from build123d import *

# Parameters (mm, degrees)
SKETCH1_W           = 19.05
SKETCH1_H           = 19.05
BOSS_EXTRUDE1_DEPTH = 19.05
SKETCH2_W           = 15.875
SKETCH2_H           = 15.875
BOSS_EXTRUDE2_DEPTH = 28.575
SKETCH3_W           = 15.875
SKETCH3_H           = 15.875
BOSS_EXTRUDE3_DEPTH = 28.575


with BuildPart() as part:
    # Sketch1 → Boss-Extrude1 (new body)
    with BuildSketch(Plane.XY):
        Rectangle(SKETCH1_W, SKETCH1_H)
    extrude(amount=BOSS_EXTRUDE1_DEPTH)

    # Sketch2 → Boss-Extrude2 (add)
    with BuildSketch(Plane(origin=(0, 9.525, 0), x_dir=(1, 0, 0), z_dir=(0, 1, 0))):
        with Locations((0, -9.525)):
            Rectangle(SKETCH2_W, SKETCH2_H)
    extrude(amount=BOSS_EXTRUDE2_DEPTH)

    # Sketch3 → Boss-Extrude3 (add)
    with BuildSketch(Plane(origin=(9.525, 0, 0), x_dir=(0, 0, -1), z_dir=(1, 0, 0))):
        with Locations((-9.525, 0)):
            Rectangle(SKETCH3_W, SKETCH3_H)
    extrude(amount=BOSS_EXTRUDE3_DEPTH)


solid = part.part
Geometry: final body of the model. Coordinates: model frame, mm. A direction names the side the tool comes from. Give positions to 0.01 mm unless a question says otherwise; leave off trailing zeros. Write each loop counter-clockwise with the first axis right and the second up, starting at its lowest first coordinate (ties: lowest second). Pieces come first, ordered by that corner, then holes.
(1) Access query for faces 1 (the flat face through (24, -7.938, 10)), 2 (the flat face through (24, 0, 17.462)), 3 (the flat face through (24, 7.938, 10)), 4 (the flat face through (0, 24, 17.462)). Directions: +Z, -Z, +X, -X, +Y, -Y. A direction counts if a zero-diameter tool reaches every point of the face in a straight line with its end or side. Return the directions, or none.
(2) Ray query, line 1 (X direction, y = 26.5, z = 12); line 2 (Z direction, x = -1.5, y = 29). Return the intervals inside material, ascending.
(3) Cut plane A-A, the plane z = 3. Return loops of the section in (x, y) (1 decimal).
(4) First-contact query: P1, Ø12.5, axis at x = -2.5, y = 17, coming from the -Z side; P2, Ø3, axis at y = 16.5, z = 3, coming from the -X side; P3, Ø4, axis at x = 29, y = -3.5, coming from the +Z side. Flat tips, straight axial feed; report the tip coordinate or a pass-through.
(5) Cut plane D-D, the plane x = 28. Return loops of the section in (y, z).
Values follow:
1. face 1: +Z, -Z, +X, -Y
1. face 2: +Z, +X, +Y, -Y
1. face 3: +Z, -Z, +X, +Y
1. face 4: +Z, +X, -X, +Y
2. line 1: x = -7.94 to 7.94
2. line 2: z = 1.59 to 17.46
3. outline: (-9.5, -9.5) - (9.5, -9.5) - (9.5, -7.9) - (38.1, -7.9) - (38.1, 7.9) - (9.5, 7.9) - (9.5, 9.5) - (7.9, 9.5) - (7.9, 38.1) - (-7.9, 38.1) - (-7.9, 9.5) - (-9.5, 9.5) - close
4. P1: stops at z = 1.59
4. P2: stops at x = -7.94
4. P3: stops at z = 17.46
5. outline: (-7.94, 1.59) - (7.94, 1.59) - (7.94, 17.46) - (-7.94, 17.46) - close
